from build123d import *

# Parameters (mm, degrees)
BOSS_EXTRUDE1_DEPTH = 6.35
SKETCH3_W           = 30
SKETCH3_H           = 6.35
BOSS_EXTRUDE2_DEPTH = 80


with BuildPart() as part:
    # Sketch2 → Boss-Extrude1 (new body)
    with BuildSketch(Plane(origin=(0, 0, 0), x_dir=(1, 0, 0), z_dir=(0, 1, 0))):
        with BuildLine():
            ThreePointArc((0, -470), (-332.340187158, -332.340187158), (-470, 0))
            Line((-470, 0), (-500, 0))
            ThreePointArc((-500, 0), (-353.553390593, -353.553390593), (0, -500))
            Line((0, -500), (0, -470))
        make_face()
    extrude(amount=BOSS_EXTRUDE1_DEPTH)

    # Sketch3 → Boss-Extrude2 (add)
    with BuildSketch(Plane(origin=(0, 0, 0), x_dir=(-1, 0, 0), z_dir=(0, 0, -1))):
        with Locations((485, 3.175)):
            Rectangle(SKETCH3_W, SKETCH3_H)
    extrude(amount=BOSS_EXTRUDE2_DEPTH)

    # Split1
    split(bisect_by=Plane(origin=(0, 0, 301), x_dir=(-1, 0, 0), z_dir=(0, 0, -1)), keep=Keep.BOTTOM)


solid = part.part
Can you work these out from the model? Positions are in its coordinate system, mm. Coordinates: 2 decimals unless noted, no trailing zeros. Write each loop counter-clockwise with the first axis right and the second up, starting at its lowest first coordinate (ties: lowest second). Pieces come first, ordered by that corner, then holes. Notation, with made-up numbers: (-10, 66.5) -> (33, 66.5) arc R29 ccw to (33, 87.5) -> close; hole circle Ø2 at (74.25, 7). An arc over 180 degrees is marked (long way). Write each question's results on one line, items separated by ' | '. Start each with the question number.
Item 1: If we section it at B-B, the plane y = 3.75: Write out the boundary of the cut face in (x, z).
Item 2: I'm going to push a flat-ended pin straight in: P1, Ø3, axis at x = -285, y = 4.5, coming from the -Z side. Where does the tip first touch, or does it pass through?
Item 3: Please list where these lines run through material, in increasing order: probe 1 along Z at (x, y) = (-98, 3.5); probe 2 along Z at (x, y) = (-85.5, 6.25); probe 3 along X at (y, z) = (1.5, 378.5).
Item 4: If we section it at A-A, the plane z = 417.5: Write out the boundary of the cut face in (x, y).
Answer block:
1) outline: (-399.25, 301) -> (-360.97, 301) arc R470 cw to (0, 470) -> (0, 500) arc R500 ccw to start
2) P1: z = 372.58
3) probe 1: 459.67 to 490.3 | probe 2: 462.16 to 492.64 | probe 3: -326.71 to -278.64
4) outline: (-275.12, 0) -> (-215.86, 0) -> (-215.86, 6.35) -> (-275.12, 6.35) -> close
